```python
from build123d import *

# Parameters (mm, degrees)
F0_W     = 10
F0_H     = 10
F1_DEPTH = 10
F2_R     = 5
F3_R     = 5


with BuildPart() as f1:
    # F0 (on Front) → F1 (new body)
    with BuildSketch(Plane.XZ):
        with BuildLine():
            ThreePointArc((46.3833183951, -18.670505474), (49.0875030927, -9.5087875211), (50, 0))
            ThreePointArc((50, 0), (49.0875030927, 9.5087875211), (46.3833183951, 18.670505474))
            ThreePointArc((46.3833183951, 18.670505474), (21.2132034356, 21.2132034356), (18.670505474, 46.3833183951))
            ThreePointArc((18.670505474, 46.3833183951), (0, 50), (-18.670505474, 46.3833183951))
            ThreePointArc((-18.670505474, 46.3833183951), (-16.2020538097, 41.113087243), (-15.3553390593, 35.3553390593))
            ThreePointArc((-15.3553390593, 35.3553390593), (-25.8832639624, 17.7405783923), (-46.3833183951, 18.670505474))
            ThreePointArc((-46.3833183951, 18.670505474), (-50, 0), (-46.3833183951, -18.670505474))
            ThreePointArc((-46.3833183951, -18.670505474), (-25.8832639624, -17.7405783923), (-15.3553390593, -35.3553390593))
            ThreePointArc((-15.3553390593, -35.3553390593), (-16.2020538097, -41.113087243), (-18.670505474, -46.3833183951))
            ThreePointArc((-18.670505474, -46.3833183951), (0, -50), (18.670505474, -46.3833183951))
            ThreePointArc((18.670505474, -46.3833183951), (21.2132034356, -21.2132034356), (46.3833183951, -18.670505474))
        make_face()
        Rectangle(F0_W, F0_H, mode=Mode.SUBTRACT)
    extrude(amount=F1_DEPTH)

    # F2
    f2_edges = [f1.edges().sort_by_distance(p)[0] for p in [
        (-46.383318, -5, 18.670505),
        (-18.670505, -5, 46.383318),
        (46.383318, -5, 18.670505),
        (18.670505, -5, 46.383318),
    ]]
    fillet(f2_edges, radius=F2_R)

    # F3
    f3_edges = [f1.edges().sort_by_distance(p)[0] for p in [
        (-18.670505, -5, -46.383318),
        (-46.383318, -5, -18.670505),
        (18.670505, -5, -46.383318),
        (46.383318, -5, -18.670505),
    ]]
    fillet(f3_edges, radius=F3_R)


solid = f1.part
```
Part model, mm, in its own coordinate system. A direction names the side the tool comes from. Round coordinates to 2 decimals unless told otherwise and drop trailing zeros. Loops run counter-clockwise (first coordinate to the right, second up) from the corner with the lowest first, then second, coordinate; pieces in that order, holes last.
Item 1: 3-axis set-ups, long thin cutter, end or side, ignore diameter. For faces 4 (the face through (-1, 0, 12)), 5 (the face through (5, -5, 0)): which of +Z, -Z, +X, -X, +Y, -Y reach the whole face in a straight line?
Item 2: Drill centre lines: line 1 (Z direction, x = -0.5, y = -8.75); line 2 (Z direction, x = -34.5, y = -1.75). Where is each one in solid material? Low to high.
Item 3: Cut at B-B, the plane z = -9.5. Give the cut face in (x, y).
Item 4: Cut at A-A, the plane x = -39. Give the cut face in (y, z), then the cut area to 3 significant figures.
Item 5: Drop flat-ended pins along their axis: P1, Ø4, axis at x = -32, y = -7, coming from the -Z side; P2, Ø6, axis at y = -6.5, z = -15, coming from the +X side; P3, Ø6, axis at y = -4.5, z = -16, coming from the +X side. Give the stop position or say it passes through.
Item 6: Mould opens along X. For faces 1 (the face through (20.99, -4.93, -21.44)), 2 (the face through (0, -5, -50)), 3 (the face through (-50, -5, 0)) say: +X half, -X half, draft (parallel to the pull), parting line (faces both ways), or undercut.
A:
1. face 4: +Z, -Z, +X, -X, +Y
1. face 5: +Y, -Y
2. line 1: z = -50 to -5, 5 to 50
2. line 2: z = -15.37 to 15.37
3. outline: (-49.09, -10) - (49.09, -10) - (49.09, 0) - (-49.09, 0) - close
4. outline: (-10, -15.69) - (0, -15.69) - (0, 15.69) - (-10, 15.69) - close
4. area: 314 mm2
5. P1: stops at z = -16.09
5. P2: stops at x = 48.54
5. P3: stops at x = 48.28
6. face 1: undercut
6. face 2: parting line
6. face 3: -X half
